Input: part model. Units: mm. Frame: model coordinates. Round coordinates to 2 decimals unless told otherwise and drop trailing zeros. Loops run counter-clockwise (first coordinate to the right, second up) from the corner with the lowest first, then second, coordinate; pieces in that order, holes last. Notation, with made-up numbers: (80, -17) - (127, -17) arc R20 ccw to (127, -11) - close; hole circle Ø4 at (-5.5, -34). An arc over 180 degrees is marked (long way). One line per question, with ' | ' between items. Start each with the question number.
Item 1: Section A-A, the plane y = -40.5. Return loops of the section in (x, z), plus the area to 3 significant figures.
Item 2: Material intervals for line 1 along Y through (x, z) = (0, 4.05); line 2 along Y through (x, z) = (0.25, 3.6); line 3 along Z through (x, y) = (0, -41.25), sorted ascending.
Item 3: Draft query along X for faces 1 (the face through (2.5, -13, 2)), 2 (the face through (0, -47.273, 1)), 3 (the face through (0.195, -42.203, 1.621)), 4 (the face through (-0.02, -36.826, 2.655)). Return one class per face: pulls with the +X half, pulls with the -X half, needs draft (parallel to the pull), parting line crosses it, or undercut.
Item 4: Section B-B, the plane z = 0.8. Return loops of the section in (x, y), plus the area to 3 significant figures.
```python
from build123d import *

# Parameters (mm, degrees)
F0_R     = 0.9
F1_DEPTH = 5
F3_D     = 1.8
F3_DEPTH = 10
F3_TIP   = 0.5407745571


with BuildPart() as f1:
    # F0 (on Top) → F1 (new body)
    with BuildSketch(Plane.XY):
        with BuildLine():
            ThreePointArc((2.5, 21.7272822881), (2.2071067812, 22.4343890692), (1.5, 22.7272822881))
            Line((1.5, 22.7272822881), (-1.5, 22.7272822881))
            ThreePointArc((-1.5, 22.7272822881), (-2.2071067812, 22.4343890692), (-2.5, 21.7272822881))
            Line((-2.5, 21.7272822881), (-2.5, -47.2727177119))
            Line((-2.5, -47.2727177119), (2.5, -47.2727177119))
            Line((2.5, -47.2727177119), (2.5, 21.7272822881))
        make_face()
        with Locations((0, 10.7272822881)):
            Circle(F0_R, mode=Mode.SUBTRACT)
        with Locations((0, 19.7272822881)):
            Circle(F0_R, mode=Mode.SUBTRACT)
    extrude(amount=F1_DEPTH)

    # F3
    with Locations(Plane.XZ.offset(47.2727177119)):
        with Locations((0, 2.5)):
            Hole(F3_D / 2, depth=F3_DEPTH)
            with Locations((0, 0, -(F3_DEPTH + F3_TIP / 2))):  # 118° drill point
                Cone(0, F3_D / 2, F3_TIP, mode=Mode.SUBTRACT)


solid = f1.part
```
Return value:
1) outline: (-2.5, 0) - (2.5, 0) - (2.5, 5) - (-2.5, 5) - close; hole circle Ø1.8 at (0, 2.5) | area: 22.5 mm2
2) line 1: -47.27 to 9.83, 11.63 to 18.83, 20.63 to 22.73 | line 2: -47.27 to 9.86, 11.59 to 18.86, 20.59 to 22.73 | line 3: 0 to 1.6, 3.4 to 5
3) face 1: pulls with the +X half | face 2: needs draft | face 3: undercut | face 4: undercut
4) outline: (-2.5, -47.27) - (2.5, -47.27) - (2.5, 21.73) arc R1 ccw to (1.5, 22.73) - (-1.5, 22.73) arc R1 ccw to (-2.5, 21.73) - close; hole circle Ø1.8 at (0, 10.73); hole circle Ø1.8 at (0, 19.73) | area: 344 mm2
